from build123d import *

# Parameters (mm, degrees)
SKETCH1_W            = 22.6
SKETCH1_H            = 11.84
BOSS_EXTRUDE1_DEPTH  = 22.7
SKETCH4_R            = 5.84
BOSS_EXTRUDE6_DEPTH  = 4.5
SKETCH12_R           = 2.335
BOSS_EXTRUDE7_DEPTH  = 2.5
SKETCH13_R           = 2.5
BOSS_EXTRUDE8_DEPTH  = 4.5
SKETCH14_W           = 11.84
SKETCH14_H           = 2.37
BOSS_EXTRUDE10_DEPTH = 4.5
SKETCH15_R           = 1
SKETCH15_W           = 1.5
SKETCH15_H           = 1
CUT_EXTRUDE3_DEPTH   = 19.7
SKETCH16_W           = 11.84
SKETCH16_H           = 2.37
BOSS_EXTRUDE11_DEPTH = 4.5
SKETCH17_R           = 1
SKETCH17_W           = 1.5
SKETCH17_H           = 1
CUT_EXTRUDE4_DEPTH   = 19.7


with BuildPart() as part:
    # Sketch1 → Boss-Extrude1 (new body)
    with BuildSketch(Plane(origin=(0, 0, 0), x_dir=(1, 0, 0), z_dir=(0, 1, 0))):
        with Locations((-34.895532414, -1.336861806)):
            Rectangle(SKETCH1_W, SKETCH1_H)
    extrude(amount=BOSS_EXTRUDE1_DEPTH)

    # Sketch4 → Boss-Extrude6 (add)
    with BuildSketch(Plane(origin=(0, 22.7, 0), x_dir=(-1, 0, 0), z_dir=(0, 1, 0))):
        with Locations((40.355532414, 1.336861806)):
            Circle(SKETCH4_R)
    extrude(amount=BOSS_EXTRUDE6_DEPTH)

    # Sketch12 → Boss-Extrude7 (add)
    with BuildSketch(Plane(origin=(0, 27.2, 0), x_dir=(-1, 0, 0), z_dir=(0, 1, 0))):
        with Locations((40.355532414, 1.336861806)):
            Circle(SKETCH12_R)
    extrude(amount=BOSS_EXTRUDE7_DEPTH)

    # Sketch13 → Boss-Extrude8 (add)
    with BuildSketch(Plane(origin=(0, 22.7, 0), x_dir=(-1, 0, 0), z_dir=(0, 1, 0))):
        with Locations((34.015532414, 1.336861806)):
            Circle(SKETCH13_R)
    extrude(amount=BOSS_EXTRUDE8_DEPTH)

    # Sketch14 → Boss-Extrude10 (add)
    with BuildSketch(Plane(origin=(-23.595532414, 0, 0), x_dir=(0, 0, -1), z_dir=(1, 0, 0))):
        with Locations((-1.336861806, 17.515)):
            Rectangle(SKETCH14_W, SKETCH14_H)
    extrude(amount=BOSS_EXTRUDE10_DEPTH)

    # Sketch15 → Cut-Extrude3 (cut, through all)
    with BuildSketch(Plane(origin=(0, 18.7, 0), x_dir=(-1, 0, 0), z_dir=(0, 1, 0))):
        with Locations((21.395532414, 1.336861806)):
            Circle(SKETCH15_R)
        with Locations((48.395532414, 1.336861806)):
            Circle(SKETCH15_R)
        with Locations((19.845532414, 1.336861806)):
            Rectangle(SKETCH15_W, SKETCH15_H)
    extrude(amount=-CUT_EXTRUDE3_DEPTH, mode=Mode.SUBTRACT)

    # Sketch16 → Boss-Extrude11 (add)
    with BuildSketch(Plane.ZY.offset(46.195532414)):
        with Locations((1.336861806, 17.515)):
            Rectangle(SKETCH16_W, SKETCH16_H)
    extrude(amount=BOSS_EXTRUDE11_DEPTH)

    # Sketch17 → Cut-Extrude4 (cut, through all)
    with BuildSketch(Plane(origin=(0, 18.7, 0), x_dir=(-1, 0, 0), z_dir=(0, 1, 0))):
        with Locations((48.295532414, 1.336861806)):
            Circle(SKETCH17_R)
        with Locations((49.945532414, 1.336861806)):
            Rectangle(SKETCH17_W, SKETCH17_H)
    extrude(amount=-CUT_EXTRUDE4_DEPTH, mode=Mode.SUBTRACT)


solid = part.part
Here's how the part is built. I have some questions about the finished solid (model axes, mm). A direction names the side the tool comes from. Round coordinates to 2 decimals unless told otherwise and drop trailing zeros. Loops run counter-clockwise (first coordinate to the right, second up) from the corner with the lowest first, then second, coordinate; pieces in that order, holes last. Notation, with made-up numbers: (84, -30) - (95, -30) arc R35 cw to (95, 2) - close; hole circle Ø9 at (20, 84.25). An arc over 180 degrees is marked (long way). One line per question, with ' | ' between items. Start each with the question number.
Q1. We'd pull the mould along X, two halves only. Please class faces 1 (the flat face through (-20, 18, 0.837)), 2 (the cylindrical face through (-42.583, 28.432, 2.038)), 3 (the cylindrical face through (-22.395, 17.532, 1.3)): +X half, -X half, draft (parallel to the pull), parting line (faces both ways), or undercut.
Q2. For faces 4 (the flat face through (-50, 18, 0.837)), 5 (the flat face through (-37, 27.2, 1)), 6 (the flat face through (-20, 18, 1.837)), 7 (the flat face through (-48, 18.7, 3)), which set-ups out of +Z, -Z, +X, -X, +Y, -Y let a thin tool reach every point of the face, with its end or its side?
Q3. I want a section at A-A (x = -48). Write out the boundary of the cut face in (y, z), then the cut area to 3 significant figures.
Q4. Please list where these lines run through material, in increasing order: line 1 (X direction, y = 20.25, z = 0.75); line 2 (Y direction, x = -37, z = -1.75); line 3 (Y direction, x = -31, z = -4). Write a range as [from, to].
Q5. I want a section at C-C (x = -42). Write out the boundary of the cut face in (y, z).
Q6. I want a section at D-D (y = 21.75). Write out the boundary of the cut face in (x, z), then the cut area to 3 significant figures.
Q7. I want a section at B-B (z = 5.25). Write out the boundary of the cut face in (x, y).
Q8. Will these pins go through, and if not, where does the flat tip stop? pin 1 (6 mm diameter, centred on x = -28, z = 4.5, fed in from +Y); pin 2 (5 mm diameter, centred on x = -22, z = 4, fed in from -Y); pin 3 (3 mm diameter, centred on y = 21, z = -1, fed in from +X); pin 4 (1.6 mm diameter, centred on x = -48.3, z = 1.34, fed in from +Y).
Response values:
1) face 1: draft | face 2: parting line | face 3: undercut
2) face 4: -X, +Y, -Y | face 5: +Y | face 6: +X, +Y, -Y | face 7: +Z, -Z, -X, +Y
3) outline: (16.33, -4.58) - (18.7, -4.58) - (18.7, 0.38) - (16.33, 0.38) - close; (16.33, 2.29) - (18.7, 2.29) - (18.7, 7.26) - (16.33, 7.26) - close | area: 23.5 mm²
4) line 1: x = [-46.2, -23.6] | line 2: y = [0, 27.2] | line 3: y = [0, 22.7]
5) outline: (0, -4.58) - (22.7, -4.58) - (22.7, -4.27) - (27.2, -4.27) - (27.2, -0.32) - (29.7, -0.32) - (29.7, 2.99) - (27.2, 2.99) - (27.2, 6.94) - (22.7, 6.94) - (22.7, 7.26) - (0, 7.26) - close
6) outline: (-46.2, -4.58) - (-23.6, -4.58) - (-23.6, 7.26) - (-46.2, 7.26) - close | area: 268 mm²
7) outline: (-50.7, 16.33) - (-46.2, 16.33) - (-46.2, 0) - (-23.6, 0) - (-23.6, 16.33) - (-19.1, 16.33) - (-19.1, 18.7) - (-23.6, 18.7) - (-23.6, 22.7) - (-36.02, 22.7) - (-36.02, 27.2) - (-44.69, 27.2) - (-44.69, 22.7) - (-46.2, 22.7) - (-46.2, 18.7) - (-50.7, 18.7) - close
8) pin 1: stops at y = 22.7 | pin 2: stops at y = 0 | pin 3: stops at x = -23.6 | pin 4: passes through
